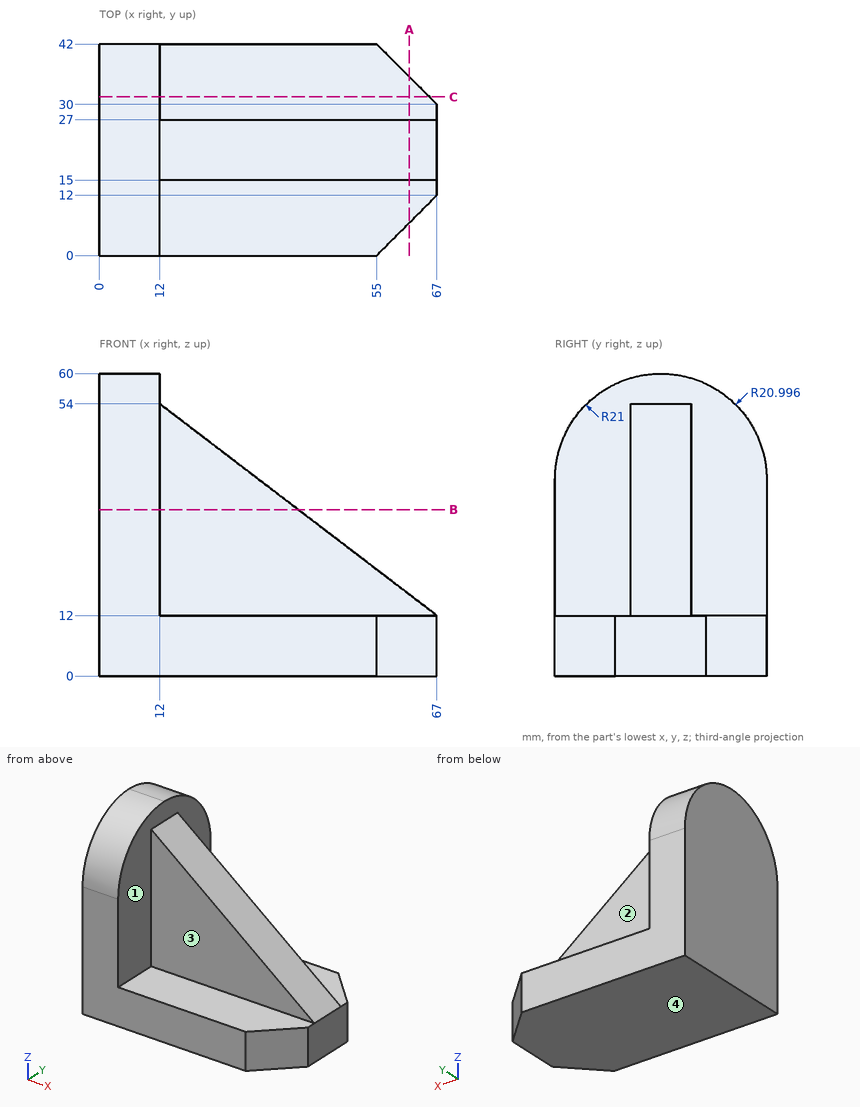
For this review, use the dimensioned drawing (mm, ordinates from the lowest corner) and the shaded views. A direction names the side the tool comes from. Coordinates: 2 decimals unless noted, no trailing zeros. Loops run counter-clockwise (first coordinate to the right, second up) from the corner with the lowest first, then second, coordinate; pieces in that order, holes last. Notation, with made-up numbers: (68, 20.25) -> (75, 20.25) arc R34 ccw to (75, 54.25) -> close; hole circle Ø7 at (18.25, 0). An arc over 180 degrees is marked (long way). Return JSON: item names as keys, results as strings. Group by question number.
(1) Tool access review of the marked faces 1, 2, 3 and 4: name each direction out of +Z, -Z, +X, -X, +Y, -Y from which nothing blocks a thin tool from reaching the whole face with its end or side.
(2) Consider section B-B, the plane z = 33. Give the boundary of the cut face in (x, y).
(3) Consider section C-C, the plane y = 31.5. Give the boundary of the cut face in (x, z), plus the area to 3 significant figures.
(4) Consider section A-A, the plane x = 61.5. Give the boundary of the cut face in (y, z), plus the area to 3 significant figures.
(5) For pin 1 Ø21 at (x, z) = (49.5, 31.5) entering from +Y; pin 2 Ø7.5 at (x, y) = (46, 10.5) entering from +Z; pin 3 Ø6 at (x, y) = (17, 18) entering from +Z; pin 4 Ø10 at (x, y) = (39, 13.5) entering from -Z, all flat-tipped, find the tip position at first contact; note any pin that passes through.
(6) To check wall thickness, follow L1, parallel to X at y = 9, z = 42; L2, parallel to Y at x = 14, z = 51. State the ranges of each line that lie inside material, in increasing order.
Results below:
{
 "1": {"face 1": "+Z, +X", "face 2": "+Z, +X, +Y", "face 3": "+Z, +X, -Y", "face 4": "-Z, +X, -X, +Y, -Y"},
 "2": {"outline": "(0, 0) -> (12, 0) -> (12, 15) -> (39.5, 15) -> (39.5, 27) -> (12, 27) -> (12, 42) -> (0, 42) -> close"},
 "3": {"outline": "(0, 0) -> (65.5, 0) -> (65.5, 12) -> (12, 12) -> (12, 57.19) -> (0, 57.19) -> close", "area": "1,330 mm2"},
 "4": {"outline": "(6.5, 0) -> (35.5, 0) -> (35.5, 12) -> (27, 12) -> (27, 16.2) -> (15, 16.2) -> (15, 12) -> (6.5, 12) -> close", "area": "398 mm2"},
 "5": {"pin 1": "stops at y = 27", "pin 2": "stops at z = 12", "pin 3": "stops at z = 52.47", "pin 4": "stops at z = 0"},
 "6": {"L1": "x = 0 to 12", "L2": "y = 15 to 27"}
}
